Input: part model. Units: mm. Frame: model coordinates. Round coordinates to 2 decimals unless told otherwise and drop trailing zeros. Loops run counter-clockwise (first coordinate to the right, second up) from the corner with the lowest first, then second, coordinate; pieces in that order, holes last. Notation, with made-up numbers: M 38.25,-16.5 L 94.25,-16.5 A13 ccw 94.25,3.5 Z; hole C 5,61 d3. An arc over 180 degrees is marked long. Return JSON: item names as keys, results as strings. Group by question number.
1) Section D-D (x = 17). Output: boundary loops of the cut face in (y, z), plus the area to 3 significant figures.
2) Material intervals for line 1 (X direction, y = 3.5, z = 14); line 2 (X direction, y = 4.25, z = 31.75); line 3 (X direction, y = 1, z = 2), sorted ascending. Write a range as from..to.
3) Section B-B (y = 4.5). Count the separate pieces of the cut face and the enclosed holes in it, plus the area to 3 significant figures.
4) Contact query for a flat-ended pin moving along its axis: P1, Ø2, axis at x = -14, z = 14, coming from the +Y side. Output: stop coordinate, or through.
5) Section A-A (z = 17). Output: boundary loops of the cut face in (x, y).
6) Section C-C (z = 31.75). Output: boundary loops of the cut face in (x, y).
from build123d import *

# Parameters (mm, degrees)
SKETCH1_W           = 50.8
SKETCH1_H           = 76.2
SKETCH1_R           = 1.3
SKETCH1_R_2         = 1.4
SKETCH1_R_3         = 2.4892
SKETCH1_W_2         = 22.5
SKETCH1_H_2         = 22.5
BOSS_EXTRUDE1_DEPTH = 6.35
FILLET1_R           = 3.175
FILLET2_R           = 1.905
FILLET3_R           = 0.79375


with BuildPart() as part:
    # Sketch1 → Boss-Extrude1 (new body)
    with BuildSketch(Plane(origin=(0, 0, 0), x_dir=(1, 0, 0), z_dir=(0, 1, 0))):
        Rectangle(SKETCH1_W, SKETCH1_H)
        with Locations(Location((-17, 17, 0), (0, 0, 270))):
            Circle(SKETCH1_R, mode=Mode.SUBTRACT)
        with Locations(Location((-17, -17, 0), (0, 0, 270))):
            Circle(SKETCH1_R, mode=Mode.SUBTRACT)
        with Locations(Location((17, -17, 0), (0, 0, 270))):
            Circle(SKETCH1_R, mode=Mode.SUBTRACT)
        with Locations(Location((17, 17, 0), (0, 0, 270))):
            Circle(SKETCH1_R, mode=Mode.SUBTRACT)
        with Locations(Location((-14, 14, 0), (0, 0, 270))):
            Circle(SKETCH1_R_2, mode=Mode.SUBTRACT)
        with Locations(Location((14, 14, 0), (0, 0, 270))):
            Circle(SKETCH1_R_2, mode=Mode.SUBTRACT)
        with Locations(Location((14, -14, 0), (0, 0, 270))):
            Circle(SKETCH1_R_2, mode=Mode.SUBTRACT)
        with Locations(Location((-14, -14, 0), (0, 0, 270))):
            Circle(SKETCH1_R_2, mode=Mode.SUBTRACT)
        with Locations(Location((-12.7, 31.75, 0), (0, 0, 270))):
            Circle(SKETCH1_R_3, mode=Mode.SUBTRACT)
        with Locations(Location((0, 31.75, 0), (0, 0, 270))):
            Circle(SKETCH1_R_3, mode=Mode.SUBTRACT)
        with Locations(Location((12.7, 31.75, 0), (0, 0, 270))):
            Circle(SKETCH1_R_3, mode=Mode.SUBTRACT)
        with Locations(Location((12.7, -31.75, 0), (0, 0, 270))):
            Circle(SKETCH1_R_3, mode=Mode.SUBTRACT)
        with Locations(Location((0, -31.75, 0), (0, 0, 270))):
            Circle(SKETCH1_R_3, mode=Mode.SUBTRACT)
        with Locations(Location((-12.7, -31.75, 0), (0, 0, 270))):
            Circle(SKETCH1_R_3, mode=Mode.SUBTRACT)
        Rectangle(SKETCH1_W_2, SKETCH1_H_2, mode=Mode.SUBTRACT)
    extrude(amount=BOSS_EXTRUDE1_DEPTH)

    # Fillet1
    fillet1_edges = [part.edges().sort_by_distance(p)[0] for p in [
        (25.4, 3.175, 38.1),
        (-25.4, 3.175, 38.1),
        (-25.4, 3.175, -38.1),
        (25.4, 3.175, -38.1),
    ]]
    fillet(fillet1_edges, radius=FILLET1_R)

    # Fillet2
    fillet2_edges = [part.edges().sort_by_distance(p)[0] for p in [
        (-11.25, 3.175, -11.25),
        (-11.25, 3.175, 11.25),
        (11.25, 3.175, 11.25),
        (11.25, 3.175, -11.25),
    ]]
    fillet(fillet2_edges, radius=FILLET2_R)

    # Fillet3
    fillet3_edges = [part.edges().sort_by_distance(p)[0] for p in [
        (-10.692038418, 0, 10.692038418),
        (-10.692038418, 6.35, 10.692038418),
        (10.692038418, 0, -10.692038418),
        (10.692038418, 6.35, -10.692038418),
        (10.692038418, 0, 10.692038418),
        (10.692038418, 6.35, 10.692038418),
        (25.4, 0, 0),
        (25.4, 6.35, 0),
        (0, 0, 38.1),
        (-25.4, 0, 0),
        (0, 0, -38.1),
        (-24.47006403, 0, -37.17006403),
        (24.47006403, 0, -37.17006403),
        (-24.47006403, 0, 37.17006403),
        (24.47006403, 0, 37.17006403),
        (0, 6.35, 38.1),
        (0, 6.35, -38.1),
        (-25.4, 6.35, 0),
        (-24.47006403, 6.35, -37.17006403),
        (24.47006403, 6.35, -37.17006403),
        (-24.47006403, 6.35, 37.17006403),
        (24.47006403, 6.35, 37.17006403),
        (0, 0, -11.25),
        (0, 6.35, -11.25),
        (-11.25, 0, 0),
        (-11.25, 6.35, 0),
        (0, 0, 11.25),
        (0, 6.35, 11.25),
        (11.25, 0, 0),
        (11.25, 6.35, 0),
        (-10.692038418, 0, -10.692038418),
        (-10.692038418, 6.35, -10.692038418),
    ]]
    fillet(fillet3_edges, radius=FILLET3_R)


solid = part.part
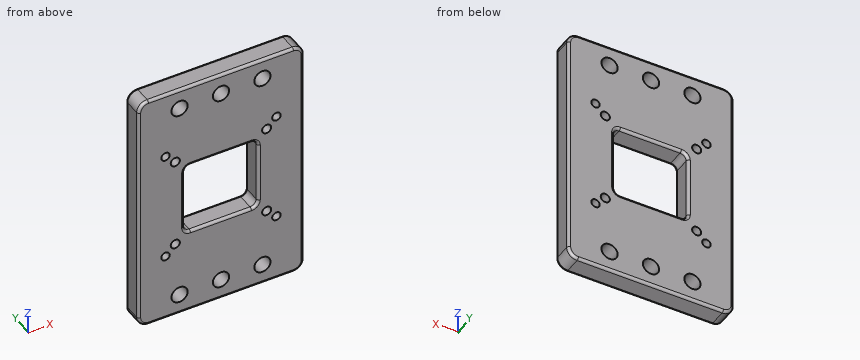
Returned:
{
 "1": {"outline": "M 0,-37.31 A0.79 ccw 0.79,-38.1 L 5.56,-38.1 A0.79 ccw 6.35,-37.31 L 6.35,-18.3 L 0,-18.3 Z; M 0,-15.7 L 6.35,-15.7 L 6.35,15.7 L 0,15.7 Z; M 0,18.3 L 6.35,18.3 L 6.35,37.31 A0.79 ccw 5.56,38.1 L 0.79,38.1 A0.79 ccw 0,37.31 Z", "area": "450 mm^2"},
 "2": {"line 1": "x = -25.4..-15.4, -12.6..12.6, 15.4..25.4", "line 2": "x = -25.4..-15.19, -10.21..-2.49, 2.49..10.21, 15.19..25.4", "line 3": "x = -25.4..-11.25, 11.25..25.4"},
 "3": {"separate pieces": "1", "enclosed holes": "15", "area": "3,200 mm^2"},
 "4": {"P1": "passes through"},
 "5": {"outline": "M -25.4,0.79 A0.79 ccw -24.61,0 L -18.3,0 L -18.3,6.35 L -24.61,6.35 A0.79 ccw -25.4,5.56 Z; M -15.7,0 L 15.7,0 L 15.7,6.35 L -15.7,6.35 Z; M 18.3,0 L 24.61,0 A0.79 ccw 25.4,0.79 L 25.4,5.56 A0.79 ccw 24.61,6.35 L 18.3,6.35 Z"},
 "6": {"outline": "M -25.4,0.79 A0.79 ccw -24.61,0 L -15.19,0 L -15.19,6.35 L -24.61,6.35 A0.79 ccw -25.4,5.56 Z; M -10.21,0 L -2.49,0 L -2.49,6.35 L -10.21,6.35 Z; M 2.49,0 L 10.21,0 L 10.21,6.35 L 2.49,6.35 Z; M 15.19,0 L 24.61,0 A0.79 ccw 25.4,0.79 L 25.4,5.56 A0.79 ccw 24.61,6.35 L 15.19,6.35 Z"}
}
